CAD build for the part. Positions are in the model's coordinates, mm. A direction names the side the tool comes from. Coordinates: 2 decimals unless noted, no trailing zeros. Order: outer loops, then holes, each group sorted by start corner. A loop starts at its lowest first (then second) coordinate and runs counter-clockwise, first axis right, second up.
from build123d import *

# Parameters (mm, degrees)
SKETCH_1_W      = 126.5
SKETCH_1_H      = 82.5
SKETCH_1_R      = 2.1
SKETCH_1_R_2    = 1.93578743
SKETCH_1_W_2    = 34.92820323
SKETCH_1_H_2    = 34.928203231
EXTRUDE_1_DEPTH = 5
SKETCH_2_W      = 126.5
SKETCH_2_H      = 82.5
EXTRUDE_2_DEPTH = 20
FILLET_1_R      = 10
CHAMFER_1_SIZE  = 3
SKETCH_3_W      = 46.92820323
SKETCH_3_H      = 46.337518094
SKETCH_3_W_2    = 40.92820323
SKETCH_3_H_2    = 40.928203231
EXTRUDE_3_DEPTH = 20
CHAMFER_2_SIZE  = 2
CHAMFER_2_SIZE2 = 19.028728908
EXTRUDE_4_DEPTH = 10


with BuildPart() as part:
    # Эскиз1 → Бобышка-Вытянуть1 (new body)
    with BuildSketch(Plane(origin=(0, 77.195974268, 0), x_dir=(1, 0, 0), z_dir=(0, 1, 0))):
        with Locations((64.808980694, -89.523129836)):
            Rectangle(SKETCH_1_W, SKETCH_1_H)
        with Locations(Location((24.808980694, -59.523129836, 0), (0, 0, 180))):
            Circle(SKETCH_1_R, mode=Mode.SUBTRACT)
        with Locations(Location((104.808980694, -59.523129836, 0), (0, 0, 180))):
            Circle(SKETCH_1_R, mode=Mode.SUBTRACT)
        with Locations(Location((104.808980694, -119.523129836, 0), (0, 0, 180))):
            Circle(SKETCH_1_R_2, mode=Mode.SUBTRACT)
        with Locations(Location((24.808980694, -119.523129836, 0), (0, 0, 180))):
            Circle(SKETCH_1_R, mode=Mode.SUBTRACT)
        with Locations((64.808980694, -89.523129837)):
            Rectangle(SKETCH_1_W_2, SKETCH_1_H_2, mode=Mode.SUBTRACT)
    extrude(amount=EXTRUDE_1_DEPTH)

    # Эскиз2 → Бобышка-Вытянуть2 (add)
    with BuildSketch(Plane(origin=(0, 82.195974268, 0), x_dir=(1, 0, 0), z_dir=(0, 1, 0))):
        with Locations((64.808980694, -89.523129836)):
            Rectangle(SKETCH_2_W, SKETCH_2_H)
        with BuildLine():
            ThreePointArc((18.350983106, -65.791643787), (21.426820016, -51.182806752), (33.808980694, -59.523129836))
            Line((33.808980694, -59.523129836), (49.308980694, -53.898129836))
            Line((49.308980694, -53.898129836), (80.308980694, -53.898129836))
            Line((80.308980694, -53.898129836), (95.808980694, -59.523129836))
            ThreePointArc((95.808980694, -59.523129836), (104.808980694, -50.523129836), (113.808980694, -59.523129836))
            ThreePointArc((113.808980694, -59.523129836), (113.149303778, -62.905290515), (111.266978282, -65.791643787))
            Line((111.266978282, -65.791643787), (120.933980694, -74.523129836))
            Line((120.933980694, -74.523129836), (120.933980694, -104.523129836))
            Line((120.933980694, -104.523129836), (111.266978282, -113.254615886))
            ThreePointArc((111.266978282, -113.254615886), (113.149303778, -116.140969158), (113.808980694, -119.523129836))
            ThreePointArc((113.808980694, -119.523129836), (104.808980694, -128.523129836), (95.808980694, -119.523129836))
            Line((95.808980694, -119.523129836), (80.308980694, -125.148129836))
            Line((80.308980694, -125.148129836), (49.308980694, -125.148129836))
            Line((49.308980694, -125.148129836), (33.808980694, -119.523129836))
            ThreePointArc((33.808980694, -119.523129836), (21.426820016, -127.86345292), (18.350983106, -113.254615886))
            Line((18.350983106, -113.254615886), (8.683980694, -104.523129836))
            Line((8.683980694, -104.523129836), (8.683980694, -74.523129836))
            Line((8.683980694, -74.523129836), (18.350983106, -65.791643787))
        make_face(mode=Mode.SUBTRACT)
    extrude(amount=EXTRUDE_2_DEPTH)

    # Скругление1
    fillet_1_edges = [part.edges().sort_by_distance(p)[0] for p in [
        (18.350983106, 92.195974268, 65.791643787),
        (33.808980694, 92.195974268, 59.523129836),
        (95.808980694, 92.195974268, 59.523129836),
        (111.266978282, 92.195974268, 65.791643787),
        (111.266978282, 92.195974268, 113.254615886),
        (95.808980694, 92.195974268, 119.523129836),
        (33.808980694, 92.195974268, 119.523129836),
        (18.350983106, 92.195974268, 113.254615886),
    ]]
    fillet(fillet_1_edges, radius=FILLET_1_R)

    # Фаска1
    chamfer_1_edges = [part.edges().sort_by_distance(p)[0] for p in [
        (64.808980694, 82.195974268, 72.059028221),
        (47.344879079, 82.195974268, 89.523129836),
        (64.808980694, 82.195974268, 106.987231452),
        (82.273082309, 82.195974268, 89.523129836),
    ]]
    chamfer(chamfer_1_edges, length=CHAMFER_1_SIZE)

    # Эскиз3 → Бобышка-Вытянуть3 (add)
    with BuildSketch(Plane(origin=(0, 82.195974268, 0), x_dir=(1, 0, 0), z_dir=(0, 1, 0))):
        with Locations((64.808980694, -89.227787268)):
            Rectangle(SKETCH_3_W, SKETCH_3_H)
        with Locations((64.808980694, -89.523129837)):
            Rectangle(SKETCH_3_W_2, SKETCH_3_H_2, mode=Mode.SUBTRACT)
    extrude(amount=EXTRUDE_3_DEPTH)

    # Фаска2
    chamfer_2_edges = [part.edges().sort_by_distance(p)[0] for p in [
        (64.808980694, 102.195974268, 69.059028221),
        (44.344879079, 102.195974268, 89.523129836),
        (64.808980694, 102.195974268, 109.987231452),
        (85.273082309, 102.195974268, 89.523129836),
    ]]
    chamfer_2_side = [part.faces().sort_by_distance(p)[0] for p in [
        (64.808980694, 102.195974268, 66.718529688),
    ]]
    chamfer(chamfer_2_edges, length=CHAMFER_2_SIZE, length2=CHAMFER_2_SIZE2, reference=chamfer_2_side[0])

    # Эскиз4 → Бобышка-Вытянуть4 (add)
    with BuildSketch(Plane(origin=(0, 102.195974268, 0), x_dir=(1, 0, 0), z_dir=(0, 1, 0))):
        Polygon((1.558980694, -48.273129836), (1.558980694, -68.273129836), (6.558980694, -68.273129836), (11.558980694, -56.273129836), (11.558980694, -48.273129836), align=None)
        Polygon((128.058980694, -48.273129836), (118.058980694, -48.273129836), (118.058980694, -56.273129836), (123.058980694, -68.273129836), (128.058980694, -68.273129836), align=None)
        Polygon((128.058980694, -130.773129836), (118.058980694, -130.773129836), (118.058980694, -122.773129836), (123.058980694, -110.773129836), (128.058980694, -110.773129836), align=None)
        Polygon((1.558980694, -130.773129836), (11.558980694, -130.773129836), (11.558980694, -122.773129836), (6.558980694, -110.773129836), (1.558980694, -110.773129836), align=None)
    extrude(amount=EXTRUDE_4_DEPTH)


solid = part.part
1) Slice it at B-B (z = 91). List the corners of the cut face in (x, y), plus the area to 3 significant figures.
2) Slice it at A-A (y = 105.5). List the corners of the cut face in (x, z).
3) Slice it at D-D (y = 88). Give the number of separate pieces and of enclosed holes in the cut face, plus the area to 3 significant figures.
4) Pin check, flat tip, straight feed: P1, Ø1, axis at x = 98, z = 60.5, coming from the +Y side. Stop position of the tip, or through.
5) Slice it at C-C (x = 61). List the corners of the cut face in (y, z).
6) Which spindle directions (+Z, -Z, +X, -X, +Y, -Y) get a long thin tool onto all of the face, cutting with end or side? Do faces 4 (the flat face through (4, 107, 110.773)), 5 (the cylindrical face through (103.68, 79.661, 61.294)), 6 (the flat face through (64.494, 92.548, 68.073)). Say none if no direction does.
7) Two-plate mould, pull along Z, no slides. Class faces 1 (the cylindrical face through (36.676, 92.336, 56.682)), 2 (the flat face through (124, 112.196, 58)), 3 (the flat face through (64, 91, 130.773)): released by +Z, released by -Z, zero draft, split by the parting line, or undercut.
8) Drill centre lines: probe 1 along X at (y, z) = (101, 77.5); probe 2 along Z at (x, y) = (79, 82.5); probe 3 along X at (y, z) = (99.5, 108.5). Where is each one in solid material? Low to high.
Worked out:
1. outline: (1.56, 77.2) - (47.34, 77.2) - (47.34, 79.2) - (44.34, 82.2) - (44.34, 83.17) - (42.34, 102.2) - (41.34, 102.2) - (41.34, 82.2) - (8.68, 82.2) - (8.68, 102.2) - (1.56, 102.2) - close; (82.27, 77.2) - (128.06, 77.2) - (128.06, 102.2) - (120.93, 102.2) - (120.93, 82.2) - (88.27, 82.2) - (88.27, 102.2) - (87.27, 102.2) - (85.27, 83.17) - (85.27, 82.2) - (82.27, 79.2) - close
1. area: 816 mm2
2. outline: (1.56, 48.27) - (11.56, 48.27) - (11.56, 56.27) - (6.56, 68.27) - (1.56, 68.27) - close; (1.56, 110.77) - (6.56, 110.77) - (11.56, 122.77) - (11.56, 130.77) - (1.56, 130.77) - close; (118.06, 48.27) - (128.06, 48.27) - (128.06, 68.27) - (123.06, 68.27) - (118.06, 56.27) - close; (118.06, 122.77) - (123.06, 110.77) - (128.06, 110.77) - (128.06, 130.77) - (118.06, 130.77) - close
3. separate pieces: 2
3. enclosed holes: 2
3. area: 3,370 mm2
4. P1: stops at y = 82.2
5. outline: (77.2, 48.27) - (102.2, 48.27) - (102.2, 53.9) - (82.2, 53.9) - (82.2, 66.06) - (102.2, 66.06) - (102.2, 67.06) - (83.17, 69.06) - (82.2, 69.06) - (79.2, 72.06) - (77.2, 72.06) - close; (77.2, 106.99) - (79.2, 106.99) - (82.2, 109.99) - (83.17, 109.99) - (102.2, 111.99) - (102.2, 112.4) - (82.2, 112.4) - (82.2, 125.15) - (102.2, 125.15) - (102.2, 130.77) - (77.2, 130.77) - close
6. face 4: +X, -X, +Y
6. face 5: +Y, -Y
6. face 6: +Y
7. face 1: undercut
7. face 2: zero draft
7. face 3: released by +Z
8. probe 1: x = 1.56 to 8.68, 41.34 to 42.47, 87.15 to 88.27, 120.93 to 128.06
8. probe 2: z = 48.27 to 53.9, 66.06 to 69.06, 109.99 to 112.4, 125.15 to 130.77
8. probe 3: x = 1.56 to 13.08, 41.34 to 42.63, 86.99 to 88.27, 116.54 to 128.06
